Geometry: see drawing. Coordinates: mm, zero at the bounding-box minimum. A direction names the side the tool comes from. Round coordinates to 2 decimals unless told otherwise and drop trailing zeros. Write each loop counter-clockwise with the first axis right and the second up, starting at its lowest first coordinate (ties: lowest second). Pieces come first, ordered by that corner, then holes. Notation, with made-up numbers: M 38,25.5 L 97,25.5 A9 cw 97,29.5 Z; hole C -19.75,61 d1. An arc over 180 degrees is marked long. Write each question's results on one line, items separated by ' | '. Start each with the question number.
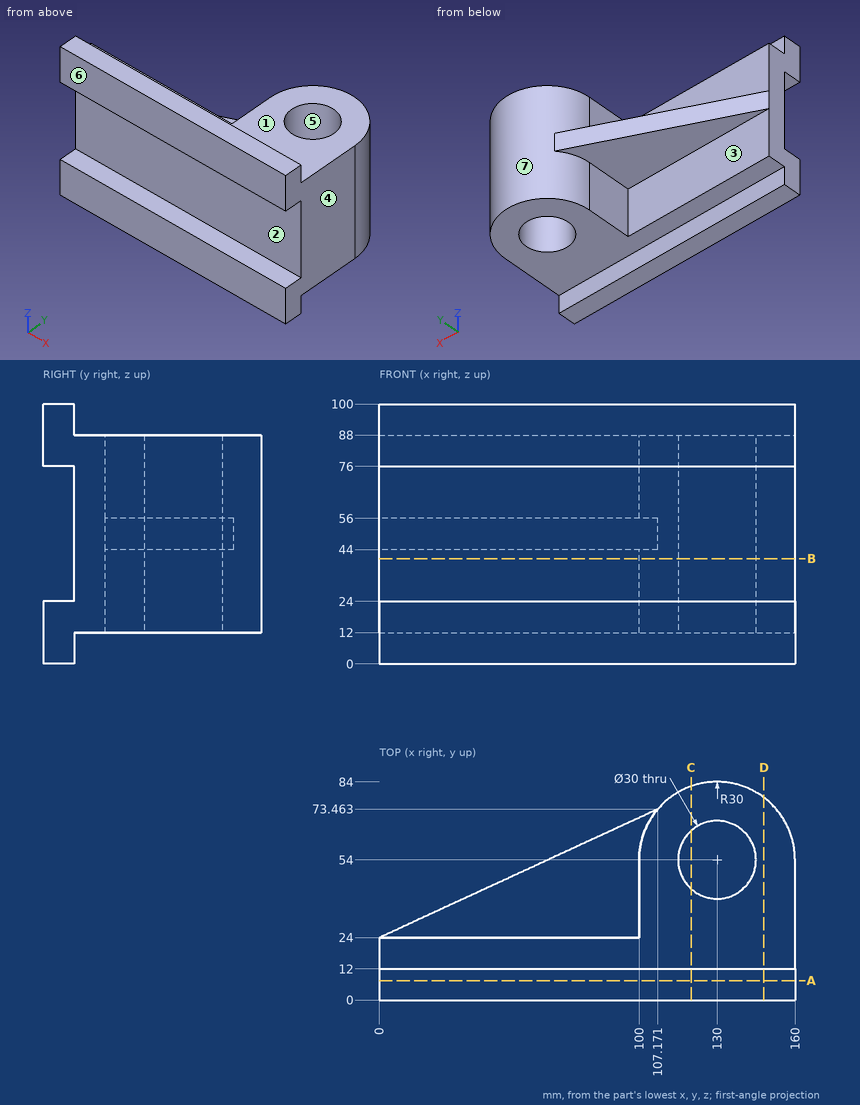
1. Cut plane A-A on y = 7.5. Output: boundary loops of the cut face in (x, z).
2. Access query for the marked faces 1, 2 and 3. Directions: +Z, -Z, +X, -X, +Y, -Y. A direction counts if a zero-diameter tool reaches every point of the face in a straight line with its end or side. Return the directions, or none.
3. Line query: L1, parallel to Y at x = 130, z = 40.5; L2, parallel to Z at x = 113, y = 8.5; L3, parallel to Y at x = 129.5, z = 23 (1 decimal). Output: solid intervals per line, ascending. Write a range as from..to.
4. Contact query for flat-ended pins moving along their axis: P1, Ø2, axis at x = 100, y = 62, coming from the +Z side; P2, Ø9.5, axis at x = 35.5, z = 24.5, coming from the +Y side; P3, Ø13, axis at x = 46.5, z = 4, coming from the +Y side. Output: stop coordinate, or through.
5. Cut plane B-B on z = 40.5. Output: boundary loops of the cut face in (x, y).
6. Cut plane D-D on x = 148. Output: boundary loops of the cut face in (y, z), and give its area (3 significant figures).
7. Draft query along Y for the marked faces 4, 5, 6 and 7. Return one class per face: +Y half, -Y half, draft (parallel to the pull), parting line (faces both ways), or undercut.
8. Cut plane C-C on x = 120. Output: boundary loops of the cut face in (y, z) (1 decimal), and give its area (3 significant figures).
Answers follow:
1) outline: M 0,0 L 160,0 L 160,24 L 0,24 Z; M 0,76 L 160,76 L 160,100 L 0,100 Z
2) face 1: +Z, +X, -X, +Y | face 2: +X, -X, -Y | face 3: -Z, -X, +Y
3) L1: y = 12..39, 69..84 | L2: z = 0..24, 76..100 | L3: y = 0..39, 69..84
4) P1: stops at z = 56 | P2: stops at y = 24 | P3: stops at y = 12
5) outline: M 0,12 L 160,12 L 160,54 A30 ccw 100,54 L 100,24 L 0,24 Z; hole C 130,54 d30
6) outline: M 0,0 L 12,0 L 12,12 L 78,12 L 78,88 L 12,88 L 12,100 L 0,100 L 0,76 L 12,76 L 12,24 L 0,24 Z | area: 5,590 mm2
7) face 4: draft | face 5: undercut | face 6: -Y half | face 7: +Y half
8) outline: M 0,0 L 12,0 L 12,12 L 42.8,12 L 42.8,88 L 12,88 L 12,100 L 0,100 L 0,76 L 12,76 L 12,24 L 0,24 Z; M 65.2,12 L 82.3,12 L 82.3,88 L 65.2,88 Z | area: 4,220 mm2
